from build123d import *

# Parameters (mm, degrees)
F0_W     = 264.16
F0_H     = 2.54
F1_DEPTH = 88.9
F3_DEPTH = 114.3


with BuildPart() as f1:
    # F0 (on Front) → F1 (new body)
    with BuildSketch(Plane.XZ):
        with Locations((-132.08, 1.27)):
            Rectangle(F0_W, F0_H)
        Polygon((0, 2.54), (0, 0), (2.54, 0), (2.54, 101.6), (0, 101.6), align=None)
        Polygon((-266.7, 0), (-264.16, 0), (-264.16, 2.54), (-264.16, 101.6), (-266.7, 101.6), align=None)
    extrude(amount=F1_DEPTH)

    # F2 (on face) → F3 (join)
    with BuildSketch(Plane(origin=(0, 0, 0), x_dir=(-1, 0, 0), z_dir=(0, 1, 0))):
        Polygon((266.7, 2.54), (264.16, 2.54), (0, 2.54), (-2.54, 2.54), (-2.54, 0), (266.7, 0), align=None)
    extrude(amount=-F3_DEPTH)


solid = f1.part
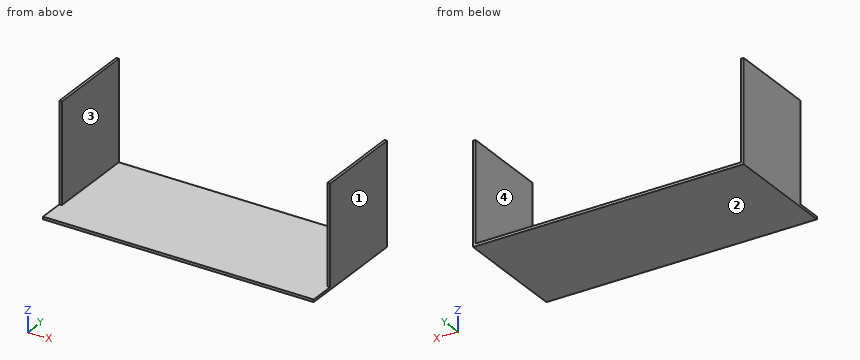
Verification items for the finished model (mm, model axes). Face numbers are marked on the shaded views. Round coordinates to 2 decimals unless told otherwise and drop trailing zeros. Loops run counter-clockwise (first coordinate to the right, second up) from the corner with the lowest first, then second, coordinate; pieces in that order, holes last. Notation, with made-up numbers: (28.25, 75.25) - (78.25, 75.25) arc R23 cw to (78.25, 107.25) - close; hole circle Ø1 at (5.25, -5.5). An arc over 180 degrees is marked (long way). Use a Markdown table: item, result. Add a question column.
1. Release check for a two-part mould opening along X. For the marked faces 1, 2, 3 and 4 record: released by +X, released by -X, zero draft, split by the parting line, or undercut.
2. Thickness scan on probe 1 along X at (y, z) = (-33.5, 26); probe 2 along Z at (x, y) = (-75, -56). Record the ranges inside material, lowest first. Write a range as [from, to].
3. Section check A-A, the plane z = 8. Record the boundary of the cut face in (x, y), plus the area to 3 significant figures.
4. Section check D-D, the plane y = -94. Record the boundary of the cut face in (x, z).
5. Section check B-B, the plane y = -65.5. Record the boundary of the cut face in (x, z).
6. Gauge pin test, flat ends, axial feed: pin 1 (2 mm diameter, centred on x = 1, z = 47, fed in from -Y); pin 2 (5 mm diameter, centred on x = -217, y = -30.5, fed in from +Z). Record the tip position at first contact, or that the pin passes through.
7. Section check C-C, the plane x = -66.5. Record the boundary of the cut face in (y, z).
Checks:
| question | item | result |
|---|---|---|
| 1 | face 1 | released by +X |
| 1 | face 2 | zero draft |
| 1 | face 3 | undercut |
| 1 | face 4 | undercut |
| 2 | probe 1 | x = [-266.7, -264.16], [0, 2.54] |
| 2 | probe 2 | z = [0, 2.54] |
| 3 | outline | (-266.7, -88.9) - (-264.16, -88.9) - (-264.16, 0) - (-266.7, 0) - close; (0, -88.9) - (2.54, -88.9) - (2.54, 0) - (0, 0) - close |
| 3 | area | 452 mm^2 |
| 4 | outline | (-266.7, 0) - (2.54, 0) - (2.54, 2.54) - (-266.7, 2.54) - close |
| 5 | outline | (-266.7, 0) - (2.54, 0) - (2.54, 101.6) - (0, 101.6) - (0, 2.54) - (-264.16, 2.54) - (-264.16, 101.6) - (-266.7, 101.6) - close |
| 6 | pin 1 | stops at y = -88.9 |
| 6 | pin 2 | stops at z = 2.54 |
| 7 | outline | (-114.3, 0) - (0, 0) - (0, 2.54) - (-114.3, 2.54) - close |
